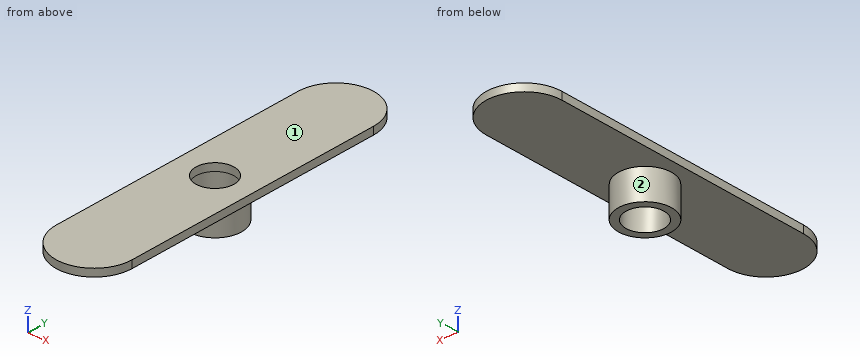
```python
from build123d import *

# Parameters (mm, degrees)
SKETCH_R      = 2.5
PAD_DEPTH     = 1
SKETCH001_R   = 3.5
SKETCH001_R_2 = 2.5
PAD001_DEPTH  = 4


with BuildPart() as part:
    # Sketch → Pad (new body)
    with BuildSketch(Plane.XY):
        with BuildLine():
            ThreePointArc((5, 17.5), (1.3e-05, 22.5), (-5, 17.500026))
            Line((-5, 17.500026), (-5, -17.5))
            ThreePointArc((-5, -17.5), (0, -22.5), (5, -17.5))
            Line((5, 17.5), (5, -17.5))
        make_face()
        Circle(SKETCH_R, mode=Mode.SUBTRACT)
    extrude(amount=-PAD_DEPTH)

    # Sketch001 (on Face7 of Pad) → Pad001 (join)
    with BuildSketch(Plane(origin=(0, 0, -1), x_dir=(1, 0, 0), z_dir=(0, 0, -1))):
        Circle(SKETCH001_R)
        Circle(SKETCH001_R_2, mode=Mode.SUBTRACT)
    extrude(amount=PAD001_DEPTH)


solid = part.part
```
Input: part model. Units: mm. Frame: model coordinates. Face numbers are marked on the shaded views. A direction names the side the tool comes from. Give positions to 0.01 mm unless a question says otherwise; leave off trailing zeros. Loops run counter-clockwise (first coordinate to the right, second up) from the corner with the lowest first, then second, coordinate; pieces in that order, holes last. Notation, with made-up numbers: M 48,36.25 L 53,36.25 A24 ccw 53,55.25 Z; hole C 23.5,79 d4. An arc over 180 degrees is marked long. Answer as CSV lines item,"result". Start each with the question number.
1. Reachability of the marked faces 1 and 2 from +Z, -Z, +X, -X, +Y, -Y: full face, straight path, thin tool, end or side. Return the list, or none.
2. Line query: L1, parallel to Y at x = 0, z = -2.4; L2, parallel to Y at x = 0, z = -0.4. Output: solid intervals per line, ascending.
3. Section B-B on z = -0.5. Return loops of the section in (x, y).
4. Pin query (flat end, axial travel): P1, Ø1.5, axis at y = 5, z = -3, coming from the -X side; P2, Ø3, axis at x = -3, z = -1.5, coming from the +Y side; P3, Ø1, axis at x = -1.5, z = -3.5, coming from the +Y side. Return the tip coordinate at first contact, or that it passes through.
5. Section C-C on y = -9. Return loops of the section in (x, z), plus the area to 3 significant figures.
6. Section A-A on x = 0. Return loops of the section in (y, z), plus the area to 3 significant figures.
7. Section D-D on z = -3.45. Return loops of the section in (x, y), plus the area to 3 significant figures.
Computed values:
1,face 1,"+Z, +X, -X, +Y, -Y"
1,face 2,"-Z"
2,L1,"y = -3.5 to -2.5, 2.5 to 3.5"
2,L2,"y = -22.5 to -2.5, 2.5 to 22.5"
3,outline,"M -5,-17.5 A5 ccw 5,-17.5 L 5,17.5 A5 ccw -5,17.5 Z; hole C 0,0 d5"
4,P1,"passes through"
4,P2,"stops at y = 22.24"
4,P3,"stops at y = 3.35"
5,outline,"M -5,-1 L 5,-1 L 5,0 L -5,0 Z"
5,area,"10.0 mm²"
6,outline,"M -22.5,-1 L -3.5,-1 L -3.5,-5 L -2.5,-5 L -2.5,0 L -22.5,0 Z; M 2.5,-5 L 3.5,-5 L 3.5,-1 L 22.5,-1 L 22.5,0 L 2.5,0 Z"
6,area,"48.0 mm²"
7,outline,"C 0,0 d7; hole C 0,0 d5"
7,area,"18.8 mm²"
